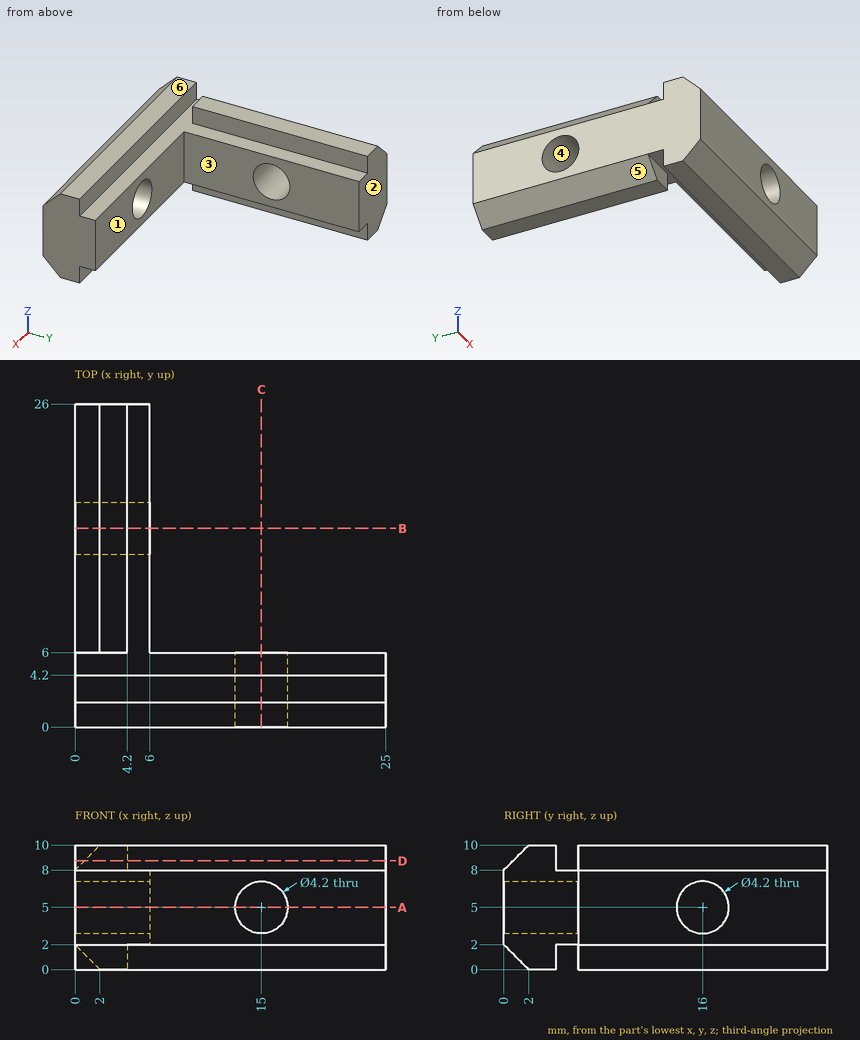
Study the drawing (mm; zero at the part's minimum x, y, z) and answer. A direction names the side the tool comes from. Coordinates: 2 decimals unless noted, no trailing zeros. Loops run counter-clockwise (first coordinate to the right, second up) from the corner with the lowest first, then second, coordinate; pieces in that order, holes last. Notation, with made-up numbers: (-15, 13) -> (22, 13) arc R14 cw to (22, 25) -> close; hole circle Ø7 at (-15, -20). An arc over 180 degrees is marked (long way). Write item = value, one per line. Start each with the question number.
1) For the marked faces 1 and 2, determine the directions among +Z, -Z, +X, -X, +Y, -Y from which every point of the face is accessible in a straight line to the end or side of a thin tool.
2) The part is cut by section B-B, the plane y = 16. Determine the outline of the cut face in (x, z), plus the area to 3 significant figures.
3) Given P1, Ø2, axis at x = 13.5, z = 0.5, coming from the +Y side; P2, Ø4, axis at y = 6.5, z = 3, coming from the +X side; P3, Ø1, axis at x = 1.5, z = 1, coming from the -Y side; P4, Ø5, axis at y = 16, z = 5.5, coming from the +X side, each flat-ended and moving along its own axis, determine where each tip first touches the part or whether it passes through.
4) The mould has two halves that part along Z. Classify the marked faces 3, 4, 5 and 6: pulls with the +Z half, pulls with the -Z half, needs draft (parallel to the pull), parting line crosses it, or undercut.
5) The part is cut by section A-A, the plane z = 5. Determine the outline of the cut face in (x, y).
6) Find the intervals of material crossed by L1, parallel to Y at x = 22.5, z = 3.75; L2, parallel to Z at x = 15, y = 1.45; L3, parallel to X at y = 3, z = 6.75, in increasing order. Write a range as from..to.
7) The part is cut by section D-D, the plane z = 8.75. Determine the outline of the cut face in (x, y).
Result:
q1.face_1 = +Z, -Z, +X, +Y
q1.face_2 = +Z, -Z, +X, -X, +Y
q2.outline = (0, 2) -> (2, 0) -> (4.2, 0) -> (4.2, 2) -> (6, 2) -> (6, 2.9) -> (0, 2.9) -> close; (0, 7.1) -> (6, 7.1) -> (6, 8) -> (4.2, 8) -> (4.2, 10) -> (2, 10) -> (0, 8) -> close
q2.area = 23.6 mm²
q3.P1 = 4.2
q3.P2 = 25
q3.P3 = 0.5
q3.P4 = 6
q4.face_3 = needs draft
q4.face_4 = undercut
q4.face_5 = pulls with the -Z half
q4.face_6 = pulls with the +Z half
q5.outline = (0, 0) -> (12.9, 0) -> (12.9, 6) -> (6, 6) -> (6, 13.9) -> (0, 13.9) -> close; (0, 18.1) -> (6, 18.1) -> (6, 26) -> (0, 26) -> close; (17.1, 0) -> (25, 0) -> (25, 6) -> (17.1, 6) -> close
q6.L1 = 0..6
q6.L2 = 0.55..2.9, 7.1..9.45
q6.L3 = 0..13.84, 16.16..25
q7.outline = (0, 0.75) -> (25, 0.75) -> (25, 4.2) -> (0, 4.2) -> close; (0.75, 6) -> (4.2, 6) -> (4.2, 26) -> (0.75, 26) -> close
